Part model, mm, in its own coordinate system. A direction names the side the tool comes from. Round coordinates to 2 decimals unless told otherwise and drop trailing zeros. Write each loop counter-clockwise with the first axis right and the second up, starting at its lowest first coordinate (ties: lowest second). Pieces come first, ordered by that corner, then holes. Notation, with made-up numbers: M 70.5,59 L 119.5,59 A24 cw 119.5,85 Z; hole C 59.25,36 d10. An arc over 180 degrees is marked long. Answer as a JSON object with one key per item and string values. Group by question number.
1. Two-plate mould, pull along X, no slides. Class faces 6 (the face through (-9.386, 1, -33)), 7 (the face through (-2, 7, -47)), 8 (the face through (-1.688, 8.619, -37.594)): +X half, -X half, draft (parallel to the pull), parting line (faces both ways), or undercut.
2. Band-saw the part on B-B, the plane x = 3.5. Write the cut outline in (y, z).
3. Band-saw the part on D-D, the plane x = -4.25. Write the cut outline in (y, z), plus the area to 3 significant figures.
4. Drill centre lines: line 1 (Z direction, x = -2.5, y = 3); line 2 (Z direction, x = 3.5, y = 3); line 3 (Y direction, x = -4.5, z = -37.5). Where is each one in solid material? Low to high. Write a range as from..to.
5. Which spindle directions (+Z, -Z, +X, -X, +Y, -Y) get a long thin tool onto all of the face, cutting with end or side? Do faces 1 (the face through (1.97, 5.51, -47.11)), 2 (the face through (-5.5, 5.31, -19.11)), 3 (the face through (-2, 4, -20.098)), 4 (the face through (-1.666, 9.395, -38.094)), 5 (the face through (-2, 7, -19)). Say none if no direction does.
6. Drop flat-ended pins along their axis: pin 1 (1.4 mm diameter, centred on x = -6.39, y = 4.5, fed in from +Z); pin 2 (1 mm diameter, centred on x = 0.5, z = -19, fed in from +Y); pin 3 (1.4 mm diameter, centred on x = 2.61, y = 4.5, fed in from -Z). Give the stop position or say it passes through.
7. Band-saw the part on A-A, the plane y = 4.5. Write the cut outline in (x, z), plus the area to 3 significant figures.
8. Band-saw the part on C-C, the plane x = 1.75. Write the cut outline in (y, z).
from build123d import *

# Parameters (mm, degrees)
ESQUISSE1_W             = 15
ESQUISSE1_H             = 30
BOSS_EXTRU_1_DEPTH      = 2
ESQUISSE4_W             = 15
ESQUISSE4_H             = 2
BOSS_EXTRU_3_DEPTH      = 5
D_GAGEMENT_M21_D        = 2.4
ESQUISSE2_R             = 5
BOSS_EXTRU_2_DEPTH      = 15
ESQUISSE3_R             = 4.5
ENL_V_MAT_EXTRU_3_DEPTH = 52.870421487


with BuildPart() as part:
    # Esquisse1 → Boss.-Extru.1 (new body)
    with BuildSketch(Plane(origin=(0, 0, 0), x_dir=(1, 0, 0), z_dir=(0, 1, 0))):
        with Locations((-1.885547836, 33.098358778)):
            Rectangle(ESQUISSE1_W, ESQUISSE1_H)
    extrude(amount=BOSS_EXTRU_1_DEPTH)

    # Esquisse4 → Boss.-Extru.3 (add)
    with BuildSketch(Plane(origin=(0, 2, 0), x_dir=(1, 0, 0), z_dir=(0, 1, 0))):
        with Locations((-1.885547836, 47.098358778)):
            Rectangle(ESQUISSE4_W, ESQUISSE4_H)
        with Locations((-1.885547836, 19.098358778)):
            Rectangle(ESQUISSE4_W, ESQUISSE4_H)
    extrude(amount=BOSS_EXTRU_3_DEPTH)

    # Dégagement M21 (through all)
    with Locations(Plane.XY.offset(-18.098358778)):
        with Locations((-6.385547836, 4.5), (2.614452164, 4.5)):
            Hole(D_GAGEMENT_M21_D / 2)

    # Esquisse2 → Boss.-Extru.2 (add)
    with BuildSketch(Plane(origin=(0, 2, 0), x_dir=(1, 0, 0), z_dir=(0, 1, 0))):
        with Locations(Location((-1.885547836, 33.098358778, 0), (0, 0, 270))):
            Circle(ESQUISSE2_R)
    extrude(amount=BOSS_EXTRU_2_DEPTH)

    # Esquisse3 → Enlèv. mat.-Extru.3 (cut, through all)
    with BuildSketch(Plane(origin=(0, 17, 0), x_dir=(1, 0, 0), z_dir=(0, 1, 0))):
        with Locations(Location((-1.885547836, 33.098358778, 0), (0, 0, 270))):
            Circle(ESQUISSE3_R)
    extrude(amount=-ENL_V_MAT_EXTRU_3_DEPTH, mode=Mode.SUBTRACT)


solid = part.part
Worked answers:
{
 "1": {"face 6": "-X half", "face 7": "draft", "face 8": "undercut"},
 "2": {"outline": "M 0,-48.1 L 3.69,-48.1 L 3.69,-46.1 L 2,-46.1 L 2,-20.1 L 3.69,-20.1 L 3.69,-18.1 L 0,-18.1 Z; M 5.31,-48.1 L 7,-48.1 L 7,-46.1 L 5.31,-46.1 Z; M 5.31,-20.1 L 7,-20.1 L 7,-18.1 L 5.31,-18.1 Z"},
 "3": {"outline": "M 0,-48.1 L 7,-48.1 L 7,-46.1 L 2,-46.1 L 2,-37.5 L 17,-37.5 L 17,-36.93 L 0,-36.93 Z; M 0,-29.27 L 17,-29.27 L 17,-28.69 L 2,-28.69 L 2,-20.1 L 7,-20.1 L 7,-18.1 L 0,-18.1 Z", "area": "82.0 mm^2"},
 "4": {"line 1": "z = -48.1..-46.1, -38.06..-37.56, -28.64..-28.14, -20.1..-18.1", "line 2": "z = -48.1..-46.1, -20.1..-18.1", "line 3": "y = 0..2"},
 "5": {"face 1": "-Z", "face 2": "+Z", "face 3": "+X, -X, +Y", "face 4": "+Y", "face 5": "+Z, +X, -X, +Y"},
 "6": {"pin 1": "stops at z = -29.85", "pin 2": "stops at y = 7", "pin 3": "stops at z = -36.35"},
 "7": {"outline": "M -9.39,-48.1 L -7.59,-48.1 L -7.59,-46.1 L -9.39,-46.1 Z; M -9.39,-20.1 L -7.59,-20.1 L -7.59,-18.1 L -9.39,-18.1 Z; C -1.89,-33.1 d10; M -5.19,-48.1 L 1.41,-48.1 L 1.41,-46.1 L -5.19,-46.1 Z; M -5.19,-20.1 L 1.41,-20.1 L 1.41,-18.1 L -5.19,-18.1 Z; M 3.81,-48.1 L 5.61,-48.1 L 5.61,-46.1 L 3.81,-46.1 Z; M 3.81,-20.1 L 5.61,-20.1 L 5.61,-18.1 L 3.81,-18.1 Z; hole C -1.89,-33.1 d9", "area": "55.7 mm^2"},
 "8": {"outline": "M 0,-48.1 L 3.67,-48.1 L 3.67,-46.1 L 2,-46.1 L 2,-36.53 L 17,-36.53 L 17,-35.75 L 0,-35.75 Z; M 0,-30.45 L 17,-30.45 L 17,-29.67 L 2,-29.67 L 2,-20.1 L 3.67,-20.1 L 3.67,-18.1 L 0,-18.1 Z; M 5.33,-48.1 L 7,-48.1 L 7,-46.1 L 5.33,-46.1 Z; M 5.33,-20.1 L 7,-20.1 L 7,-18.1 L 5.33,-18.1 Z"}
}
